Design review of the part built by this model. Coordinates are the model's own, in mm. A direction names the side the tool comes from. Coordinates: 2 decimals unless noted, no trailing zeros. Order: outer loops, then holes, each group sorted by start corner. A loop starts at its lowest first (then second) coordinate and runs counter-clockwise, first axis right, second up. Notation, with made-up numbers: M 13,-39.75 L 19,-39.75 A22 ccw 19,-0.75 Z; hole C 10,52 d7. An arc over 180 degrees is marked long. Answer as a JSON object with one key per item and string values.
from build123d import *

# Parameters (mm, degrees)
SKETCH1_R           = 1.6
BOSS_EXTRUDE1_DEPTH = 4
BOSS_EXTRUDE2_DEPTH = 4
SKETCH3_R           = 6
BOSS_EXTRUDE3_DEPTH = 4
SKETCH4_R           = 2
CUT_EXTRUDE1_DEPTH  = 62.753461441
SKETCH5_W           = 50
SKETCH5_H           = 59.8
BOSS_EXTRUDE4_DEPTH = 6
SKETCH6_R           = 2.1
CUT_EXTRUDE2_DEPTH  = 6
FILLET1_R           = 4


with BuildPart() as part:
    # Sketch1 → Boss-Extrude1 (new body)
    with BuildSketch(Plane.XY):
        with BuildLine():
            Line((-15, -28), (15, -28))
            Line((15, -28), (15, 31.5))
            ThreePointArc((15, 31.5), (12.071067812, 38.571067812), (5, 41.5))
            Line((5, 41.5), (-5, 41.5))
            ThreePointArc((-5, 41.5), (-12.071067812, 38.571067812), (-15, 31.5))
            Line((-15, 31.5), (-15, -28))
        make_face()
        with Locations((-5, 34.75)):
            Circle(SKETCH1_R, mode=Mode.SUBTRACT)
        with Locations((-5, -13.85)):
            Circle(SKETCH1_R, mode=Mode.SUBTRACT)
        with Locations(Location((5, 34.75, 0), (0, 0, 180))):
            Circle(SKETCH1_R, mode=Mode.SUBTRACT)
        with Locations(Location((5, -13.85, 0), (0, 0, 180))):
            Circle(SKETCH1_R, mode=Mode.SUBTRACT)
        Polygon((-10.3, -10.3), (-0.83, -10.3), (-0.83, -16.7), (0.83, -16.7), (0.83, -10.3), (10.3, -10.3), (10.3, 31.2), (0.83, 31.2), (0.83, 37.6), (-0.83, 37.6), (-0.83, 31.2), (-10.3, 31.2), align=None, mode=Mode.SUBTRACT)
    extrude(amount=BOSS_EXTRUDE1_DEPTH)



with BuildPart() as body_2:
    # Sketch2 → Boss-Extrude2 (new body)
    with BuildSketch(Plane.XY.offset(39.2)):
        with BuildLine():
            Line((-15, -28), (15, -28))
            Line((15, -28), (15, 0))
            ThreePointArc((15, 0), (0, 15), (-15, 0))
            Line((-15, 0), (-15, -28))
        make_face()
    extrude(amount=-BOSS_EXTRUDE2_DEPTH)

    # Sketch3 → Boss-Extrude3 (add)
    with BuildSketch(Plane.XY.offset(39.2)):
        Circle(SKETCH3_R)
    extrude(amount=BOSS_EXTRUDE3_DEPTH)

    # Sketch4 → Cut-Extrude1 (cut, through all)
    with BuildSketch(Plane.XY.offset(43.2)):
        Circle(SKETCH4_R)
    extrude(amount=-CUT_EXTRUDE1_DEPTH, mode=Mode.SUBTRACT)


with BuildPart() as part_1:
    add(part.part)

    add(body_2.part)  # Boss-Extrude4 merges body 2
    # Sketch5 → Boss-Extrude4 (add)
    with BuildSketch(Plane(origin=(0, -28, 0), x_dir=(1, 0, 0), z_dir=(0, 1, 0))):
        with Locations((0, -19.3)):
            Rectangle(SKETCH5_W, SKETCH5_H)
    extrude(amount=-BOSS_EXTRUDE4_DEPTH)

    # Sketch6 → Cut-Extrude2 (cut)
    with BuildSketch(Plane.XZ.offset(34)):
        with Locations(Location((-20, 45.4, 0), (0, 0, 270))):
            Circle(SKETCH6_R)
        with Locations(Location((20, 45.4, 0), (0, 0, 90))):
            Circle(SKETCH6_R)
        with Locations(Location((20, -6.8, 0), (0, 0, 270))):
            Circle(SKETCH6_R)
        with Locations(Location((-20, -6.8, 0), (0, 0, 90))):
            Circle(SKETCH6_R)
    extrude(amount=-CUT_EXTRUDE2_DEPTH, mode=Mode.SUBTRACT)

    # Fillet1
    fillet1_edges = [part_1.edges().sort_by_distance(p)[0] for p in [
        (15, -28, 2),
        (-15, -28, 2),
        (0, -28, 0),
        (-15, -28, 37.2),
        (0, -28, 35.2),
        (15, -28, 37.2),
        (0, -28, 39.2),
        (0, -28, 4),
    ]]
    fillet(fillet1_edges, radius=FILLET1_R)


solid = part_1.part
1) Tool access review of faces 5 (the cylindrical face through (-6, 0, 41)), 6 (the flat face through (-0.83, -13, 2)), 7 (the flat face through (-5, 31.2, 2)): name each direction out of +Z, -Z, +X, -X, +Y, -Y from which nothing blocks a thin tool from reaching the whole face with its end or side.
Taken from the geometry:
{"face 5": "+Z", "face 6": "-Z", "face 7": "+Z, -Z"}
2) Add section D-D (y = 34.75). State the section outline as (x, z) points, and give its area (3 significant figures).
Taken from the geometry:
{"outline": "M -14.46,0 L -6.6,0 L -6.6,4 L -14.46,4 Z; M -3.4,0 L -0.83,0 L -0.83,4 L -3.4,4 Z; M 0.83,0 L 3.4,0 L 3.4,4 L 0.83,4 Z; M 6.6,0 L 14.46,0 L 14.46,4 L 6.6,4 Z", "area": "83.4 mm2"}
3) Add section B-B (z = -6.8). State the section outline as (x, y) points, and give its area (3 significant figures).
Taken from the geometry:
{"outline": "M -25,-34 L -22.1,-34 L -22.1,-28 L -25,-28 Z; M -17.9,-34 L 17.9,-34 L 17.9,-28 L -17.9,-28 Z; M 22.1,-34 L 25,-34 L 25,-28 L 22.1,-28 Z", "area": "250 mm2"}
4) Add section A-A (y = -13.85). State the section outline as (x, z) points, and give its area (3 significant figures).
Taken from the geometry:
{"outline": "M -15,0 L -6.6,0 L -6.6,4 L -15,4 Z; M -15,35.2 L 15,35.2 L 15,39.2 L -15,39.2 Z; M -3.4,0 L -0.83,0 L -0.83,4 L -3.4,4 Z; M 0.83,0 L 3.4,0 L 3.4,4 L 0.83,4 Z; M 6.6,0 L 15,0 L 15,4 L 6.6,4 Z", "area": "208 mm2"}
5) Mouldability with a two-part tool opening along Y and no side actions: class faces 1 (the cylindrical face through (-11.99, 38.65, 1.97)), 2 (the flat face through (0, -31, -10.6)), 3 (the flat face through (0, -16.7, 2)), 4 (the cylindrical face through (4, 36, 2)) as released by +Y, released by -Y, zero draft, split by the parting line, or undercut.
Taken from the geometry:
{"face 1": "released by +Y", "face 2": "zero draft", "face 3": "undercut", "face 4": "undercut"}
6) Add section C-C (x = 20). State the section outline as (y, z) points.
Taken from the geometry:
{"outline": "M -34,-10.6 L -28,-10.6 L -28,-8.9 L -34,-8.9 Z; M -34,-4.7 L -28,-4.7 L -28,43.3 L -34,43.3 Z; M -34,47.5 L -28,47.5 L -28,49.2 L -34,49.2 Z"}
7) To check wall thickness, follow L1, parallel to X at y = -29.7, z = 45.4; L2, parallel to Y at x = 5, z = 2; L3, parallel to Z at x = -8, y = -15.5. State the ranges of each line that lie inside material, in increasing order.
Taken from the geometry:
{"L1": "x = -25 to -22.1, -17.9 to 17.9, 22.1 to 25", "L2": "y = -34 to -15.45, -12.25 to -10.3, 31.2 to 33.15, 36.35 to 41.5", "L3": "z = 0 to 4, 35.2 to 39.2"}
8) Insertion check: pin 1 Ø15 at (x, y) = (0.5, 2.5) entering from -Z; pin 2 Ø2 at (y, z) = (5.5, 2) entering from -X; pin 3 Ø3 at (x, y) = (-4.5, -8) entering from +Z. Each pin has a flat end and moves straight along its axis. Give the tip position at first contact, or say it passes through.
Taken from the geometry:
{"pin 1": "stops at z = 35.2", "pin 2": "stops at x = -15", "pin 3": "stops at z = 39.2"}
